Autodesk Inventor part; units mm, degrees
ref_plane "YZ Plane" through (0, 0, 0) normal (1, 0, 0) x (0, 1, 0)
ref_plane "XZ Plane" through (0, 0, 0) normal (0, 1, 0) x (-1, 0, 0)
ref_plane "XY Plane" through (0, 0, 0) normal (0, 0, 1) x (1, 0, 0)
sketch "Boceto1" plane through (0, 0, 0) normal (0, 0, 1) x (1, 0, 0)
  line L0 (-40, -40) -> (40, -40)
  line L1 (40, -40) -> (40, 40)
  line L2 (40, 40) -> (-40, 40)
  line L3 (-40, 40) -> (-40, -40)
  line L4 (-40, -40) -> (40, 40) construction
  line L5 (40, -40) -> (-40, 40) construction
  point P0 (0, 0)
  dimension "d0" = 80
  dimension "d1" = 80
extrude "Extrusión1" add sketch "Boceto1" along normal blind 90
sketch "Boceto2" plane through (0, 0, 90) normal (0, 0, 1) x (1, 0, 0)
  circle A0 centre (0, 0) radius 25
  circle A1 centre (0, 0) radius 22.5
  dimension "d4" = 50
  dimension "d5" = 45
extrude "Extrusión2" add sketch "Boceto2" along normal blind 50
sketch "Boceto3" plane through (0, 0, 0) normal (0, 0, -1) x (-1, 0, 0)
  line L0 (-35, -35) -> (35, -35)
  line L1 (35, -35) -> (35, 35)
  line L2 (35, 35) -> (-35, 35)
  line L3 (-35, 35) -> (-35, -35)
  line L4 (-35, -35) -> (35, 35) construction
  line L5 (35, -35) -> (-35, 35) construction
  line L6 (-40, 40) -> (40, 40)
  line L7 (-40, -40) -> (-40, 40)
  circle A0 centre (-37.5, 37.5) radius 1.9
  circle A1 centre (37.5, 37.5) radius 1.9
  circle A2 centre (37.5, -37.5) radius 1.9
  circle A3 centre (-37.5, -37.5) radius 1.9
  point P0 (0, 0)
  dimension "d9" = 70
sketch "Boceto4" plane through (0, 0, 0) normal (0, 0, -1) x (-1, 0, 0)
  point P0 (0, 0)
extrude "Extrusión3" cut sketch "Boceto3" against normal blind 90 contours A0 | A1 | A2 | A3
sketch "Boceto5" plane through (0, 0, 90) normal (0, 0, 1) x (1, 0, 0)
  circle A0 centre (0, 0) radius 22.5
  dimension "d14" = 45
extrude "Extrusión4" add sketch "Boceto5" along normal blind 20
thread "Rosca1"
thread "Rosca2"
thread "Rosca3"
thread "Rosca4"
thread "Rosca5"
properties part number "PRACTICA 1"
Part model, mm, in its own coordinate system. A direction names the side the tool comes from. Give positions to 0.01 mm unless a question says otherwise; leave off trailing zeros. Order: outer loops, then holes, each group sorted by start corner. A loop starts at its lowest first (then second) coordinate and runs counter-clockwise, first axis right, second up. Notation, with made-up numbers: (-16, 19) - (14, 19) arc R34 ccw to (14, 52) - close; hole circle Ø7 at (-30.75, -23.75). An arc over 180 degrees is marked (long way). Use a Markdown table: item, result.
1) Flat gauge pins, fed straight in: P1, Ø3, axis at x = 37.5, y = 37.5, coming from the +Z side; P2, Ø4, axis at x = 5, y = -15.5, coming from the +Z side; P3, Ø4.5, axis at x = -37.5, y = -37.5, coming from the +Z side; P4, Ø1.5, axis at x = 14, z = 120, coming from the -Y side. Where does each tip first touch, or does it go through?
Checked values:
| item | result |
|---|---|
| P1 | through |
| P2 | z = 110 |
| P3 | z = 90 |
| P4 | y = -21.2 |
2) Saw through at C-C on y = -4. List the corners of the cut face in (x, z).
Checked values:
| item | result |
|---|---|
| outline | (-40, 0) - (40, 0) - (40, 90) - (24.68, 90) - (24.68, 140) - (22.14, 140) - (22.14, 110) - (-22.14, 110) - (-22.14, 140) - (-24.68, 140) - (-24.68, 90) - (-40, 90) - close |
3) Saw through at D-D on z = 121.5. List the corners of the cut face in (x, y).
Checked values:
| item | result |
|---|---|
| outline | circle Ø50 at (0, 0); hole circle Ø45 at (0, 0) |
4) Saw through at A-A on y = -37.5. List the corners of the cut face in (x, z), plus the area to 3 significant figures.
Checked values:
| item | result |
|---|---|
| outline | (-40, 0) - (-39.4, 0) - (-39.4, 90) - (-40, 90) - close; (-35.6, 0) - (35.6, 0) - (35.6, 90) - (-35.6, 90) - close; (39.4, 0) - (40, 0) - (40, 90) - (39.4, 90) - close |
| area | 6,520 mm² |
5) Two-plate mould, pull along Y, no slides. Class faces 1 (the flat face through (1, 40, 44)), 2 (the cylindrical face through (23.846, -7.509, 114.65)), 3 (the flat face through (-18, 18, 90)), 4 (the cylindrical face through (10.382, 19.961, 124.79)): +Y half, -Y half, draft (parallel to the pull), parting line (faces both ways), or undercut.
Checked values:
| item | result |
|---|---|
| face 1 | +Y half |
| face 2 | parting line |
| face 3 | draft |
| face 4 | undercut |
6) Saw through at B-B on x = 15.5. List the corners of the cut face in (y, z), plus the area to 3 significant figures.
Checked values:
| item | result |
|---|---|
| outline | (-40, 0) - (40, 0) - (40, 90) - (19.62, 90) - (19.62, 140) - (16.31, 140) - (16.31, 110) - (-16.31, 110) - (-16.31, 140) - (-19.62, 140) - (-19.62, 90) - (-40, 90) - close |
| area | 8,180 mm² |
7) 3-axis set-ups, long thin cutter, end or side, ignore diameter. For faces 5 (the flat face through (0, 0, 110)), 6 (the cylindrical face through (35.745, -38.228, 44.37)): which of +Z, -Z, +X, -X, +Y, -Y reach the whole face in a straight line?
Checked values:
| item | result |
|---|---|
| face 5 | +Z |
| face 6 | +Z, -Z |
8) Probe L1, parallel to Y at x = -37.5, z = 32; L2, parallel to Y at x = -37, z = 61. List the from-to ranges inside material, lowest first. Write a range as from..to.
Checked values:
| item | result |
|---|---|
| L1 | -40..-39.4, -35.6..35.6, 39.4..40 |
| L2 | -40..-39.33, -35.67..35.67, 39.33..40 |
